```python
from build123d import *

# Parameters (mm, degrees)
F0_W      = 60
F0_H      = 12.3176118359
F1_DEPTH  = 10
F2_DEPTH  = 60
F3_W      = 88
F3_H      = 98
F4_DEPTH  = 5
F5_DEPTH  = 70
F6_D      = 5.6
F6_DEPTH  = 10
F6_TIP    = 1.6824097333
F8_DEPTH  = 25
F9_W      = 88
F9_H      = 4.2
F10_DEPTH = 75.001
F12_D     = 5.6
F12_DEPTH = 10
F12_TIP   = 1.6824097333


with BuildPart() as f1:
    # F0 (on Top) → F1 (new body)
    with BuildSketch(Plane.XY):
        Polygon((-37, 40), (-30, 40), (-30, 49), (-44, 49), (-44, -49), (-30, -49), (-30, -40), (-37, -40), align=None)
        Polygon((-30, -6.1588059179), (-30, 6.1588059179), (-30, 40), (-37, 40), (-37, -40), (-30, -40), align=None)
        Rectangle(F0_W, F0_H)
        Polygon((37, -40), (37, 40), (30, 40), (30, 6.1588059179), (30, -6.1588059179), (30, -40), align=None)
        Polygon((30, 40), (37, 40), (37, -40), (30, -40), (30, -49), (44, -49), (44, 49), (30, 49), align=None)
    extrude(amount=-F1_DEPTH)

    # F2 (add): a face of the model
    f2_faces = [f1.faces().sort_by_distance(p)[0] for p in [
        (0, 0, -10),
    ]]
    extrude(f2_faces, amount=F2_DEPTH)

    # F3 (on face) → F4 (join)
    with BuildSketch(Plane(origin=(0, 0, -70), x_dir=(1, 0, 0), z_dir=(0, 0, -1))):
        Rectangle(F3_W, F3_H)
    extrude(amount=F4_DEPTH)

    # F0 (on Top) → F5 (cut, through all)
    with BuildSketch(Plane.XY):
        Rectangle(F0_W, F0_H)
    extrude(amount=-F5_DEPTH, mode=Mode.SUBTRACT)

    # F6
    with Locations(Plane.XY):
        with Locations((-37, 40), (-37, -40), (37, -40), (37, 40)):
            Hole(F6_D / 2, depth=F6_DEPTH)
            with Locations((0, 0, -(F6_DEPTH + F6_TIP / 2))):  # 118° drill point
                Cone(0, F6_D / 2, F6_TIP, mode=Mode.SUBTRACT)

    # F7 (on face) → F8 (join)
    with BuildSketch(Plane.XZ.offset(49)):
        with BuildLine():
            ThreePointArc((-17.500000122, -70), (-26.338834808, -66.3388347217), (-30, -57.5))
            Line((-30, -57.5), (-30, -70))
            Line((-30, -70), (-17.500000122, -70))
        make_face()
        with BuildLine():
            ThreePointArc((30, -57.5), (26.3388347648, -66.3388347648), (17.5, -70))
            Line((17.5, -70), (30, -70))
            Line((30, -70), (30, -57.5))
        make_face()
    extrude(amount=-F8_DEPTH)

    # F9 (on face) → F10 (cut, through all)
    with BuildSketch(Plane.XY):
        with Locations((0, 46.9)):
            Rectangle(F9_W, F9_H)
    extrude(amount=-F10_DEPTH, mode=Mode.SUBTRACT)

    # F12
    with Locations(Plane(origin=(-44, 0, 0), x_dir=(0, -1, 0), z_dir=(-1, 0, 0))):
        with Locations((5.7637224598, -23.1461717886), (39.7637224598, -23.1461717886), (5.7637224598, -65.1461717886), (39.7637224598, -65.1461717886)):
            Hole(F12_D / 2, depth=F12_DEPTH)
            with Locations((0, 0, -(F12_DEPTH + F12_TIP / 2))):  # 118° drill point
                Cone(0, F12_D / 2, F12_TIP, mode=Mode.SUBTRACT)


solid = f1.part
```
Geometry check sheet. Reference: the model listing, model coordinates, mm. A direction names the side the tool comes from. Give positions to 0.01 mm unless a question says otherwise; leave off trailing zeros. Loops run counter-clockwise (first coordinate to the right, second up) from the corner with the lowest first, then second, coordinate; pieces in that order, holes last. Notation, with made-up numbers: (-1.5, 58) - (17.5, 58) arc R12 cw to (17.5, 74) - close; hole circle Ø3 at (9, 63). An arc over 180 degrees is marked (long way). Use CSV: the item, a comma, the result in double quotes. Start each with the question number.
Q1. Scan lines: probe 1 along X at (y, z) = (-40, -4); probe 2 along Y at (x, z) = (37, -6); probe 3 along X at (y, z) = (0, -12). Record each from-to range of solid material in increasing order. Write a range as from..to.
Q2. Section check D-D, the plane z = -60.5. Record the cut outline in (x, y), and give its area (3 significant figures).
Q3. Section check C-C, the plane x = 19.5. Record the cut outline in (y, z).
Q4. Access from +Z, -Z, +X, -X, +Y, -Y to the whole of each face (thin tool, end or side, straight path). Record for faces 4 (the face through (-38.93, -6.37, -67.88)), 5 (the face through (0, -3, -70)), 6 (the face through (37.607, -42.733, -5.07)), 7 (the face through (-1, -3, -75)).
Q5. Go/stop test with flat-tipped pins: pin 1 Ø3 at (x, y) = (12.5, -33) entering from +Z; pin 2 Ø3.5 at (x, y) = (-37, -40) entering from +Z; pin 3 Ø3.5 at (y, z) = (-39.76, -65.15) entering from -X. Record where each tip stops, or that it passes through.
Q6. Release check for a two-part mould opening along Y. For faces 1 (the face through (44, -1, -37)), 2 (the face through (0, 44.8, -71)), 3 (the face through (-32.61, -5.7, -22.66)) record: +Y half, -Y half, draft (parallel to the pull), parting line (faces both ways), or undercut.
Q7. Section check A-A, the plane z = -43.5. Record the cut outline in (x, y).
Q8. Section check B-B, the plane y = 6. Record the cut outline in (x, z), and give its area (3 significant figures).
Findings below:
1,probe 1,"x = -44..-39.8, -34.2..-30, 30..34.2, 39.8..44"
1,probe 2,"y = -49..-42.8, -37.2..37.2, 42.8..44.8"
1,probe 3,"x = -44..-30, 30..44"
2,outline,"(-44, -49) - (-29.63, -49) - (-29.63, -24) - (-30, -24) - (-30, 44.8) - (-44, 44.8) - close; (29.63, -49) - (44, -49) - (44, 44.8) - (30, 44.8) - (30, -24) - (29.63, -24) - close"
2,area,"2,640 mm^2"
3,outline,"(-49, -75) - (44.8, -75) - (44.8, -70) - (-24, -70) - (-24, -69.84) - (-49, -69.84) - close"
4,face 4,"-X"
4,face 5,"+Z, +Y"
4,face 6,"+Z"
4,face 7,"-Z, +X, -X, +Y, -Y"
5,pin 1,"stops at z = -70"
5,pin 2,"stops at z = -10.63"
5,pin 3,"stops at x = -33.37"
6,face 1,"draft"
6,face 2,"+Y half"
6,face 3,"undercut"
7,outline,"(-44, -49) - (-30, -49) - (-30, 44.8) - (-44, 44.8) - close; (30, -49) - (44, -49) - (44, 44.8) - (30, 44.8) - close"
8,outline,"(-44, -75) - (44, -75) - (44, 0) - (30, 0) - (30, -70) - (-30, -70) - (-30, 0) - (-44, 0) - close"
8,area,"2,400 mm^2"
